Verification items for this drawing (mm, ordinates from the low corner). A direction names the side the tool comes from. Give positions to 0.01 mm unless a question says otherwise; leave off trailing zeros. Write each loop counter-clockwise with the first axis right and the second up, starting at its lowest first coordinate (ties: lowest second). Pieces come first, ordered by that corner, then holes. Notation, with made-up numbers: (-29, -26.75) -> (25, -26.75) arc R16 cw to (25, -11.75) -> close; hole circle Ø3 at (59, 18). An arc over 180 degrees is marked (long way). Use one line per item in the form item = value. Start each with the question number.
(1) Section check B-B, the plane z = 80.5. Record the cut outline in (x, y).
(2) Depth check by flat-ended pin: pin 1 Ø6.5 at (x, y) = (67, 67.5) entering from +Z; pin 2 Ø10 at (x, z) = (52.5, 20) entering from -Y; pin 3 Ø6.5 at (x, z) = (91, 47.5) entering from -Y. Enter the tip coordinate at first touch or a pass-through.
(3) Scan lines: L1, parallel to Z at x = 33, y = 35.5; L2, parallel to Y at x = 15, z = 54.5; L3, parallel to Y at x = 6, z = 38. Record each from-to range of solid material in increasing order.
(4) Set-up check for the marked faces 1 and 2: record each of +Z, -Z, +X, -X, +Y, -Y from which the full face is reachable in a straight line by a thin tool's end or side.
(5) Section check C-C, the plane y = 61. Record the cut outline in (x, z), plus the area to 3 significant figures.
(6) Section check A-A, the plane x = 70.5. Record the cut outline in (y, z), plus the area to 3 significant figures.
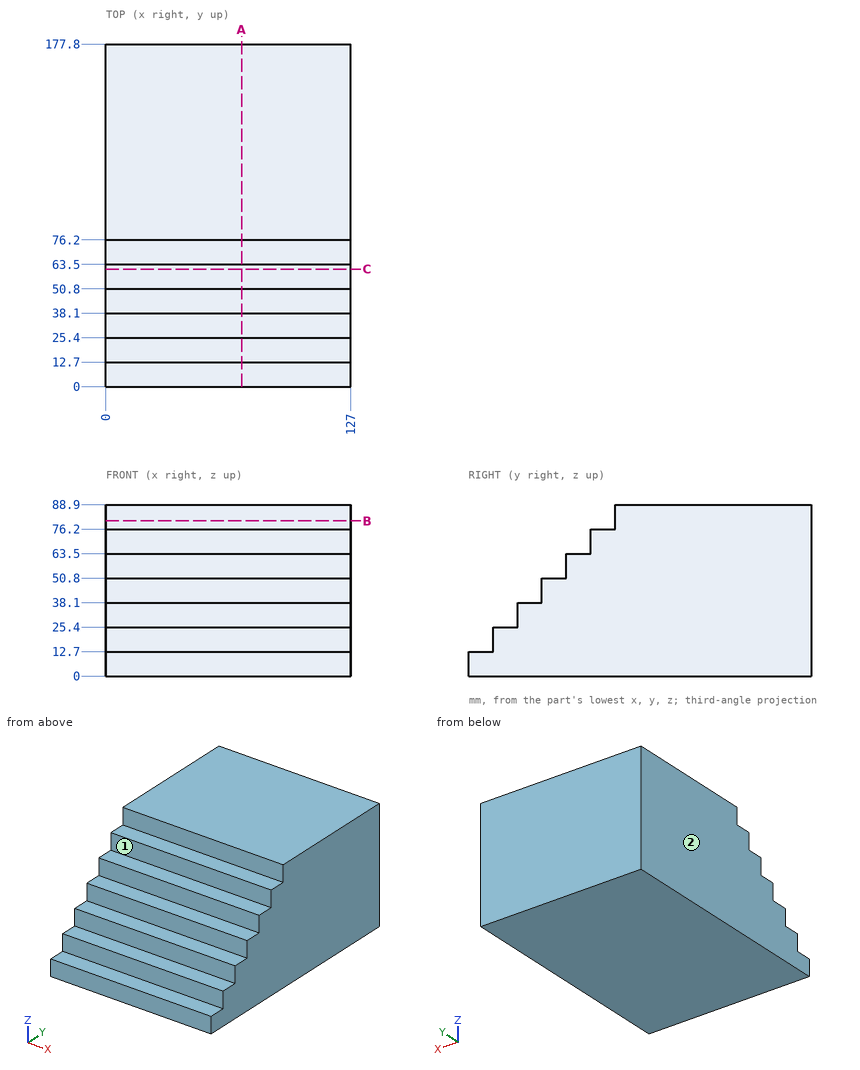
Completed:
q1.outline = (0, 76.2) -> (127, 76.2) -> (127, 177.8) -> (0, 177.8) -> close
q2.pin_1 = 76.2
q2.pin_2 = 12.7
q2.pin_3 = 38.1
q3.L1 = 0 to 38.1
q3.L2 = 50.8 to 177.8
q3.L3 = 25.4 to 177.8
q4.face_1 = +Z, +X, -X, -Y
q4.face_2 = +Z, -Z, -X, +Y, -Y
q5.outline = (0, 0) -> (127, 0) -> (127, 63.5) -> (0, 63.5) -> close
q5.area = 8,060 mm²
q6.outline = (0, 0) -> (177.8, 0) -> (177.8, 88.9) -> (76.2, 88.9) -> (76.2, 76.2) -> (63.5, 76.2) -> (63.5, 63.5) -> (50.8, 63.5) -> (50.8, 50.8) -> (38.1, 50.8) -> (38.1, 38.1) -> (25.4, 38.1) -> (25.4, 25.4) -> (12.7, 25.4) -> (12.7, 12.7) -> (0, 12.7) -> close
q6.area = 12,400 mm²
